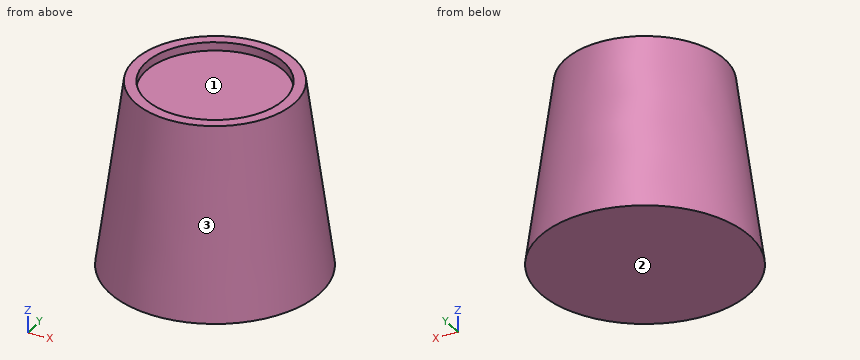
from build123d import *

# Parameters (mm, degrees)
F0_R     = 62.5
F1_DEPTH = 110
F2_SIZE2 = 109.99999
F2_SIZE  = 14.99999
F3_R     = 41
F4_DEPTH = 5


# Not quite as in the source:
# - a fillet or chamfer is up to 0.001 mm smaller than in the source, because OpenCascade refuses the exact size


with BuildPart() as f1:
    # F0 (on Top) → F1 (new body)
    with BuildSketch(Plane.XY):
        Circle(F0_R)
    extrude(amount=F1_DEPTH)

    # F2 (size 15 and 110 in the source; OpenCascade refuses exactly that, so slightly less here)
    f2_edges = [f1.edges().sort_by_distance(p)[0] for p in [
        (-62.5, 0, 110),
    ]]
    f2_side = f1.faces().sort_by_distance((0, 0, 110))[0]
    chamfer(f2_edges, length=F2_SIZE, length2=F2_SIZE2, reference=f2_side)

    # F3 (on face) → F4 (cut)
    with BuildSketch(Plane.XY.offset(110)):
        Circle(F3_R)
    extrude(amount=-F4_DEPTH, mode=Mode.SUBTRACT)


solid = f1.part
Design review of the part built by this model. Coordinates are the model's own, in mm. Face numbers are marked on the shaded views. Give positions to 0.01 mm unless a question says otherwise; leave off trailing zeros. Order: outer loops, then holes, each group sorted by start corner. A loop starts at its lowest first (then second) coordinate and runs counter-clockwise, first axis right, second up. Notation, with made-up numbers: (-3.5, 7) - (29.5, 7) arc R15 cw to (29.5, 22) - close; hole circle Ø8 at (14, -3.75). An arc over 180 degrees is marked (long way). Write item = value, one per line. Start each with the question number.
Q1. Mouldability with a two-part tool opening along X and no side actions: class the marked faces 1, 2 and 3 as released by +X, released by -X, zero draft, split by the parting line, or undercut.
Q2. We need section D-D on z = 79. State the section outline as (x, y) points.
Q3. Clearance check with flat-ended pins moving along their axes: pin 1 Ø1.5 at (y, z) = (-34.5, 87.5) entering from -X; pin 2 Ø4 at (x, z) = (16.5, 90.5) entering from +Y; pin 3 Ø6 at (x, z) = (40, 91.5) entering from -Y. State where each tip first meets the part, or that it passes through.
Q4. We need section C-C on z = 47.5. State the section outline as (x, y) points, plus the area to 3 significant figures.
Q5. To check wall thickness, follow L1, parallel to Z at x = -22.5, y = 2; L2, parallel to Y at x = 0, z = 107; L3, parallel to Y at x = 0, z = 107.9. State the ranges of each line that lie inside material, in increasing order. Write a range as from..to.
Working result:
q1.face_1 = undercut
q1.face_2 = zero draft
q1.face_3 = split by the parting line
q2.outline = circle Ø103.45 at (0, 0)
q3.pin_1 = -37.67
q3.pin_2 = 48.08
q3.pin_3 = -33.72
q4.outline = circle Ø112.05 at (0, 0)
q4.area = 9,860 mm²
q5.L1 = 0..105
q5.L2 = -47.91..-41, 41..47.91
q5.L3 = -47.79..-41, 41..47.79
